Check sheet for the modelled part. Datum: model origin and axes. Units: mm. Coordinates: 2 decimals unless noted, no trailing zeros. Order: outer loops, then holes, each group sorted by start corner. A loop starts at its lowest first (then second) coordinate and runs counter-clockwise, first axis right, second up. Notation, with made-up numbers: M 29,-39.5 L 47,-39.5 A19 cw 47,-3.5 Z; hole C -3,45.5 d11. An arc over 180 degrees is marked long. Answer in a Markdown table with one row per item. Add a question column.
from build123d import *

# Parameters (mm, degrees)
SKETCH1_W                     = 161
SKETCH1_H                     = 150
SKETCH1_W_2                   = 15.5
SKETCH1_H_2                   = 23
BOSS_EXTRUDE1_DEPTH           = 2.032
CSK_FOR_M3_SFHCS1_AT_2_COUNT  = 2
CSK_FOR_M3_SFHCS1_AT_2_PITCH  = 26.979181982
CSK_FOR_M3_SFHCS1_AT_3_COUNT  = 2
CSK_FOR_M3_SFHCS1_AT_3_PITCH  = 49.851028074
CSK_FOR_M3_SFHCS1_AT_4_COUNT  = 2
CSK_FOR_M3_SFHCS1_AT_4_PITCH  = 65.133507042
CSK_FOR_M3_SFHCS1_AT_5_COUNT  = 2
CSK_FOR_M3_SFHCS1_AT_5_PITCH  = 70.5
CSK_FOR_M3_SFHCS1_AT_6_COUNT  = 2
CSK_FOR_M3_SFHCS1_AT_6_PITCH  = 65.133507042
CSK_FOR_M3_SFHCS1_AT_7_COUNT  = 2
CSK_FOR_M3_SFHCS1_AT_7_PITCH  = 49.851028074
CSK_FOR_M3_SFHCS1_AT_8_COUNT  = 2
CSK_FOR_M3_SFHCS1_AT_8_PITCH  = 26.979181982
CSK_FOR_M3_SFHCS1_AT_9_COUNT  = 2
CSK_FOR_M3_SFHCS1_AT_9_PITCH  = 40.25
CSK_FOR_M3_SFHCS1_AT_10_COUNT = 2
CSK_FOR_M3_SFHCS1_AT_10_PITCH = 33.035019298
CSK_FOR_M3_SFHCS1_AT_11_COUNT = 2
CSK_FOR_M3_SFHCS1_AT_11_PITCH = 33.035019298
CUT_EXTRUDE1_DEPTH            = 3.032
FILLET1_R                     = 1
CSK_FOR_M3_SFHCS2_AT_2_COUNT  = 2
CSK_FOR_M3_SFHCS2_AT_2_PITCH  = 35.5
CSK_FOR_M3_SFHCS2_AT_3_COUNT  = 2
CSK_FOR_M3_SFHCS2_AT_3_PITCH  = 81.038571063
CSK_FOR_M3_SFHCS2_AT_4_COUNT  = 2
CSK_FOR_M3_SFHCS2_AT_4_PITCH  = 61.288253361
CSK_FOR_M3_SFHCS2_AT_5_COUNT  = 2
CSK_FOR_M3_SFHCS2_AT_5_PITCH  = 55.939699677
CSK_FOR_M3_SFHCS2_AT_6_COUNT  = 2
CSK_FOR_M3_SFHCS2_AT_6_PITCH  = 55.939699677
CSK_FOR_M3_SFHCS2_AT_7_COUNT  = 2
CSK_FOR_M3_SFHCS2_AT_7_PITCH  = 61.288253361
CSK_FOR_M3_SFHCS2_AT_8_COUNT  = 2
CSK_FOR_M3_SFHCS2_AT_8_PITCH  = 81.038571063
CSK_FOR_M3_SFHCS2_AT_9_COUNT  = 2
CSK_FOR_M3_SFHCS2_AT_9_PITCH  = 35.5
CSK_FOR_M3_SFHCS2_AT_10_COUNT = 2
CSK_FOR_M3_SFHCS2_AT_10_PITCH = 113.80355882
CSK_FOR_M3_SFHCS2_AT_11_COUNT = 2
CSK_FOR_M3_SFHCS2_AT_11_PITCH = 120.537338613
CSK_FOR_M3_SFHCS2_AT_12_COUNT = 2
CSK_FOR_M3_SFHCS2_AT_12_PITCH = 137.68169813
CSK_FOR_M3_SFHCS2_AT_13_COUNT = 2
CSK_FOR_M3_SFHCS2_AT_13_PITCH = 137.68169813
CSK_FOR_M3_SFHCS2_AT_14_COUNT = 2
CSK_FOR_M3_SFHCS2_AT_14_PITCH = 120.537338613
CSK_FOR_M3_SFHCS2_AT_15_COUNT = 2
CSK_FOR_M3_SFHCS2_AT_15_PITCH = 113.80355882
CSK_FOR_M3_SFHCS2_AT_16_COUNT = 2
CSK_FOR_M3_SFHCS2_AT_16_PITCH = 139.508064283
CSK_FOR_M3_SFHCS2_AT_17_COUNT = 2
CSK_FOR_M3_SFHCS2_AT_17_PITCH = 137
CSK_FOR_M3_SFHCS2_AT_18_COUNT = 2
CSK_FOR_M3_SFHCS2_AT_18_PITCH = 139.508064283


with BuildPart() as part:
    # Sketch1 → Boss-Extrude1 (new body)
    with BuildSketch(Plane(origin=(0, 0, 0), x_dir=(1, 0, 0), z_dir=(0, 1, 0))):
        with Locations((0, -1)):
            Rectangle(SKETCH1_W, SKETCH1_H)
        with Locations((-66.75, 50)):
            Rectangle(SKETCH1_W_2, SKETCH1_H_2, mode=Mode.SUBTRACT)
        with Locations((66.75, 50)):
            Rectangle(SKETCH1_W_2, SKETCH1_H_2, mode=Mode.SUBTRACT)
        with Locations((66.75, -50)):
            Rectangle(SKETCH1_W_2, SKETCH1_H_2, mode=Mode.SUBTRACT)
        with Locations((-66.75, -50)):
            Rectangle(SKETCH1_W_2, SKETCH1_H_2, mode=Mode.SUBTRACT)
    extrude(amount=BOSS_EXTRUDE1_DEPTH)

    # Sketch2 → CSK for M3 SFHCS1 (revolve, cut)
    with BuildSketch(Plane(origin=(0, 0, 35.25), x_dir=(0, 0, -1), z_dir=(1, 0, 0))):
        Polygon((0, 0), (0, 2.032), (1.6, 2.032), (1.6, 1.4), (3, 0), align=None)
    csk_for_m3_sfhcs1 = revolve(axis=Axis((0, -6.35, 35.25), (0, 1, 0)), mode=Mode.SUBTRACT)

    # CSK for M3 SFHCS1 at 2: CSK for M3 SFHCS1 ×2
    with Locations(*[Vector(0.923879533, 0, -0.382683432) * (i * CSK_FOR_M3_SFHCS1_AT_2_PITCH) for i in range(1, CSK_FOR_M3_SFHCS1_AT_2_COUNT)]):
        add(csk_for_m3_sfhcs1, mode=Mode.SUBTRACT)

    # CSK for M3 SFHCS1 at 3: CSK for M3 SFHCS1 ×2
    with Locations(*[Vector(0.707106781, 0, -0.707106781) * (i * CSK_FOR_M3_SFHCS1_AT_3_PITCH) for i in range(1, CSK_FOR_M3_SFHCS1_AT_3_COUNT)]):
        add(csk_for_m3_sfhcs1, mode=Mode.SUBTRACT)

    # CSK for M3 SFHCS1 at 4: CSK for M3 SFHCS1 ×2
    with Locations(*[Vector(0.382683432, 0, -0.923879533) * (i * CSK_FOR_M3_SFHCS1_AT_4_PITCH) for i in range(1, CSK_FOR_M3_SFHCS1_AT_4_COUNT)]):
        add(csk_for_m3_sfhcs1, mode=Mode.SUBTRACT)

    # CSK for M3 SFHCS1 at 5: CSK for M3 SFHCS1 ×2
    with Locations(*[(0, 0, -i * CSK_FOR_M3_SFHCS1_AT_5_PITCH) for i in range(1, CSK_FOR_M3_SFHCS1_AT_5_COUNT)]):
        add(csk_for_m3_sfhcs1, mode=Mode.SUBTRACT)

    # CSK for M3 SFHCS1 at 6: CSK for M3 SFHCS1 ×2
    with Locations(*[Vector(-0.382683432, 0, -0.923879533) * (i * CSK_FOR_M3_SFHCS1_AT_6_PITCH) for i in range(1, CSK_FOR_M3_SFHCS1_AT_6_COUNT)]):
        add(csk_for_m3_sfhcs1, mode=Mode.SUBTRACT)

    # CSK for M3 SFHCS1 at 7: CSK for M3 SFHCS1 ×2
    with Locations(*[Vector(-0.707106781, 0, -0.707106781) * (i * CSK_FOR_M3_SFHCS1_AT_7_PITCH) for i in range(1, CSK_FOR_M3_SFHCS1_AT_7_COUNT)]):
        add(csk_for_m3_sfhcs1, mode=Mode.SUBTRACT)

    # CSK for M3 SFHCS1 at 8: CSK for M3 SFHCS1 ×2
    with Locations(*[Vector(-0.923879533, 0, -0.382683432) * (i * CSK_FOR_M3_SFHCS1_AT_8_PITCH) for i in range(1, CSK_FOR_M3_SFHCS1_AT_8_COUNT)]):
        add(csk_for_m3_sfhcs1, mode=Mode.SUBTRACT)

    # CSK for M3 SFHCS1 at 9: CSK for M3 SFHCS1 ×2
    with Locations(*[(0, 0, -i * CSK_FOR_M3_SFHCS1_AT_9_PITCH) for i in range(1, CSK_FOR_M3_SFHCS1_AT_9_COUNT)]):
        add(csk_for_m3_sfhcs1, mode=Mode.SUBTRACT)

    # CSK for M3 SFHCS1 at 10: CSK for M3 SFHCS1 ×2
    with Locations(*[Vector(-0.131076873, 0, -0.991372207) * (i * CSK_FOR_M3_SFHCS1_AT_10_PITCH) for i in range(1, CSK_FOR_M3_SFHCS1_AT_10_COUNT)]):
        add(csk_for_m3_sfhcs1, mode=Mode.SUBTRACT)

    # CSK for M3 SFHCS1 at 11: CSK for M3 SFHCS1 ×2
    with Locations(*[Vector(0.131076873, 0, -0.991372207) * (i * CSK_FOR_M3_SFHCS1_AT_11_PITCH) for i in range(1, CSK_FOR_M3_SFHCS1_AT_11_COUNT)]):
        add(csk_for_m3_sfhcs1, mode=Mode.SUBTRACT)

    # Sketch4 → Cut-Extrude1 (cut, through all)
    with BuildSketch(Plane.XZ):
        Polygon((59, -38.5), (72.5, -35), (72.5, 35), (59, 38.5), (59, 63.5), (30.5, 76), (80.5, 76), (80.5, -74), (26, -74), (59, -69.528648916), align=None)
        Polygon((-80.5, 76), (-80.5, -74), (-26, -74), (-59, -69.528648916), (-59, -38.5), (-72.5, -35), (-72.5, 35), (-59, 38.5), (-59, 63.5), (-30.5, 76), align=None)
    extrude(amount=-CUT_EXTRUDE1_DEPTH, mode=Mode.SUBTRACT)

    # Fillet1
    fillet1_edges = [part.edges().sort_by_distance(p)[0] for p in [
        (-59, 1.016, -38.5),
        (59, 1.016, -69.528648916),
        (72.5, 1.016, -35),
        (72.5, 1.016, 35),
        (59, 1.016, 63.5),
        (30.5, 1.016, 76),
        (26, 1.016, -74),
        (-30.5, 1.016, 76),
        (-59, 1.016, 63.5),
        (-72.5, 1.016, 35),
        (-72.5, 1.016, -35),
        (-59, 1.016, -69.528648916),
        (-26, 1.016, -74),
        (59, 1.016, -38.5),
        (59, 1.016, 38.5),
        (-59, 1.016, 38.5),
    ]]
    fillet(fillet1_edges, radius=FILLET1_R)

    # Sketch5 → CSK for M3 SFHCS2 (revolve, cut)
    with BuildSketch(Plane(origin=(0, 0, 66.5), x_dir=(0, 0, -1), z_dir=(1, 0, 0))):
        Polygon((0, 0), (0, 2.032), (1.6, 2.032), (1.6, 1.4), (3, 0), align=None)
    csk_for_m3_sfhcs2 = revolve(axis=Axis((0, -6.35, 66.5), (0, 1, 0)), mode=Mode.SUBTRACT)

    # CSK for M3 SFHCS2 at 2: CSK for M3 SFHCS2 ×2
    with Locations(*[(-i * CSK_FOR_M3_SFHCS2_AT_2_PITCH, 0, 0) for i in range(1, CSK_FOR_M3_SFHCS2_AT_2_COUNT)]):
        add(csk_for_m3_sfhcs2, mode=Mode.SUBTRACT)

    # CSK for M3 SFHCS2 at 3: CSK for M3 SFHCS2 ×2
    with Locations(*[Vector(-0.851446405, 0, -0.524441626) * (i * CSK_FOR_M3_SFHCS2_AT_3_PITCH) for i in range(1, CSK_FOR_M3_SFHCS2_AT_3_COUNT)]):
        add(csk_for_m3_sfhcs2, mode=Mode.SUBTRACT)

    # CSK for M3 SFHCS2 at 4: CSK for M3 SFHCS2 ×2
    with Locations(*[Vector(-0.905556888, 0, -0.424224849) * (i * CSK_FOR_M3_SFHCS2_AT_4_PITCH) for i in range(1, CSK_FOR_M3_SFHCS2_AT_4_COUNT)]):
        add(csk_for_m3_sfhcs2, mode=Mode.SUBTRACT)

    # CSK for M3 SFHCS2 at 5: CSK for M3 SFHCS2 ×2
    with Locations(*[Vector(-0.992139756, 0, -0.125134744) * (i * CSK_FOR_M3_SFHCS2_AT_5_PITCH) for i in range(1, CSK_FOR_M3_SFHCS2_AT_5_COUNT)]):
        add(csk_for_m3_sfhcs2, mode=Mode.SUBTRACT)

    # CSK for M3 SFHCS2 at 6: CSK for M3 SFHCS2 ×2
    with Locations(*[Vector(0.992139756, 0, -0.125134744) * (i * CSK_FOR_M3_SFHCS2_AT_6_PITCH) for i in range(1, CSK_FOR_M3_SFHCS2_AT_6_COUNT)]):
        add(csk_for_m3_sfhcs2, mode=Mode.SUBTRACT)

    # CSK for M3 SFHCS2 at 7: CSK for M3 SFHCS2 ×2
    with Locations(*[Vector(0.905556888, 0, -0.424224849) * (i * CSK_FOR_M3_SFHCS2_AT_7_PITCH) for i in range(1, CSK_FOR_M3_SFHCS2_AT_7_COUNT)]):
        add(csk_for_m3_sfhcs2, mode=Mode.SUBTRACT)

    # CSK for M3 SFHCS2 at 8: CSK for M3 SFHCS2 ×2
    with Locations(*[Vector(0.851446405, 0, -0.524441626) * (i * CSK_FOR_M3_SFHCS2_AT_8_PITCH) for i in range(1, CSK_FOR_M3_SFHCS2_AT_8_COUNT)]):
        add(csk_for_m3_sfhcs2, mode=Mode.SUBTRACT)

    # CSK for M3 SFHCS2 at 9: CSK for M3 SFHCS2 ×2
    with Locations(*[(i * CSK_FOR_M3_SFHCS2_AT_9_PITCH, 0, 0) for i in range(1, CSK_FOR_M3_SFHCS2_AT_9_COUNT)]):
        add(csk_for_m3_sfhcs2, mode=Mode.SUBTRACT)

    # CSK for M3 SFHCS2 at 10: CSK for M3 SFHCS2 ×2
    with Locations(*[Vector(0.606307928, 0, -0.795229964) * (i * CSK_FOR_M3_SFHCS2_AT_10_PITCH) for i in range(1, CSK_FOR_M3_SFHCS2_AT_10_COUNT)]):
        add(csk_for_m3_sfhcs2, mode=Mode.SUBTRACT)

    # CSK for M3 SFHCS2 at 11: CSK for M3 SFHCS2 ×2
    with Locations(*[Vector(0.46043824, 0, -0.887691741) * (i * CSK_FOR_M3_SFHCS2_AT_11_PITCH) for i in range(1, CSK_FOR_M3_SFHCS2_AT_11_COUNT)]):
        add(csk_for_m3_sfhcs2, mode=Mode.SUBTRACT)

    # CSK for M3 SFHCS2 at 12: CSK for M3 SFHCS2 ×2
    with Locations(*[Vector(0.403103686, 0, -0.915154314) * (i * CSK_FOR_M3_SFHCS2_AT_12_PITCH) for i in range(1, CSK_FOR_M3_SFHCS2_AT_12_COUNT)]):
        add(csk_for_m3_sfhcs2, mode=Mode.SUBTRACT)

    # CSK for M3 SFHCS2 at 13: CSK for M3 SFHCS2 ×2
    with Locations(*[Vector(-0.403103686, 0, -0.915154314) * (i * CSK_FOR_M3_SFHCS2_AT_13_PITCH) for i in range(1, CSK_FOR_M3_SFHCS2_AT_13_COUNT)]):
        add(csk_for_m3_sfhcs2, mode=Mode.SUBTRACT)

    # CSK for M3 SFHCS2 at 14: CSK for M3 SFHCS2 ×2
    with Locations(*[Vector(-0.46043824, 0, -0.887691741) * (i * CSK_FOR_M3_SFHCS2_AT_14_PITCH) for i in range(1, CSK_FOR_M3_SFHCS2_AT_14_COUNT)]):
        add(csk_for_m3_sfhcs2, mode=Mode.SUBTRACT)

    # CSK for M3 SFHCS2 at 15: CSK for M3 SFHCS2 ×2
    with Locations(*[Vector(-0.606307928, 0, -0.795229964) * (i * CSK_FOR_M3_SFHCS2_AT_15_PITCH) for i in range(1, CSK_FOR_M3_SFHCS2_AT_15_COUNT)]):
        add(csk_for_m3_sfhcs2, mode=Mode.SUBTRACT)

    # CSK for M3 SFHCS2 at 16: CSK for M3 SFHCS2 ×2
    with Locations(*[Vector(0.290305799, 0, -0.956933928) * (i * CSK_FOR_M3_SFHCS2_AT_16_PITCH) for i in range(1, CSK_FOR_M3_SFHCS2_AT_16_COUNT)]):
        add(csk_for_m3_sfhcs2, mode=Mode.SUBTRACT)

    # CSK for M3 SFHCS2 at 17: CSK for M3 SFHCS2 ×2
    with Locations(*[(0, 0, -i * CSK_FOR_M3_SFHCS2_AT_17_PITCH) for i in range(1, CSK_FOR_M3_SFHCS2_AT_17_COUNT)]):
        add(csk_for_m3_sfhcs2, mode=Mode.SUBTRACT)

    # CSK for M3 SFHCS2 at 18: CSK for M3 SFHCS2 ×2
    with Locations(*[Vector(-0.290305799, 0, -0.956933928) * (i * CSK_FOR_M3_SFHCS2_AT_18_PITCH) for i in range(1, CSK_FOR_M3_SFHCS2_AT_18_COUNT)]):
        add(csk_for_m3_sfhcs2, mode=Mode.SUBTRACT)


solid = part.part
1. Section check B-B on x = -46. Enter the section's corners in (y, z).
2. Release check for a two-part mould opening along X. For faces 1 (the flat face through (-1, 2.032, 0)), 2 (the conical face through (0, 1, -3)) record: released by +X, released by -X, zero draft, split by the parting line, or undercut.
3. Scan lines: line 1 (X direction, y = 1.65, z = -40.5); line 2 (X direction, y = 1.7, z = -23.5); line 3 (Z direction, x = -26.5, y = 0.55). Record each from-to range of solid material in increasing order.
4. Section check A-A on y = 0.6. State how many separate pieces and enclosed holes the cut face has, then the cut area to 3 significant figures.
5. Go/stop test with flat-tipped pins: pin 1 Ø3.5 at (x, z) = (-69, -24) entering from -Y; pin 2 Ø2.5 at (x, z) = (-55.5, -40.5) entering from +Y; pin 3 Ø1 at (y, z) = (1, -48.5) entering from -X; pin 4 Ø4 at (x, z) = (55.5, 59.5) entering from -Y. Record where each tip stops, or that it passes through.
Result sheet:
| question | item | result |
|---|---|---|
| 1 | outline | M 0,-71.29 L 2.03,-71.29 L 2.03,69.2 L 0,69.2 Z |
| 2 | face 1 | zero draft |
| 2 | face 2 | undercut |
| 3 | line 1 | -59 to -57.1, -53.9 to 53.9, 57.1 to 59 |
| 3 | line 2 | -72.5 to -70.52, -67.48 to -25.65, -24.2 to 24.2, 25.65 to 67.48, 70.52 to 72.5 |
| 3 | line 3 | -73.93 to -26.8, -23.05 to 23.05, 26.8 to 76 |
| 4 | separate pieces | 1 |
| 4 | enclosed holes | 29 |
| 4 | area | 18,700 mm^2 |
| 5 | pin 1 | y = 1.25 |
| 5 | pin 2 | through |
| 5 | pin 3 | x = -59 |
| 5 | pin 4 | y = 1 |
